Input: part model. Units: mm. Frame: model coordinates. Face numbers are marked on the shaded views. A direction names the side the tool comes from. Coordinates: 2 decimals unless noted, no trailing zeros. Write each loop counter-clockwise with the first axis right and the second up, starting at its lowest first coordinate (ties: lowest second). Pieces come first, ordered by that corner, then holes. Notation, with made-up numbers: M 59,62.5 L 74,62.5 A30 ccw 74,91.5 Z; hole C 17,46.5 d8. An arc over 180 degrees is marked long. Use one line per item in the form item = value.
from build123d import *

# Parameters (mm, degrees)
SKETCH_1_R          = 4
EXTRUDE_1_DEPTH     = 5.5
SKETCH_2_R          = 5
EXTRUDE_2_DEPTH     = 1.5
SKETCH_3_R          = 2.75
CUT_EXTRUDE_1_DEPTH = 2
SKETCH_4_R          = 1.5
CUT_EXTRUDE_2_DEPTH = 8
CHAMFER_1_SIZE      = 0.2
CHAMFER_2_SIZE      = 0.2
CHAMFER_3_SIZE      = 0.2
CHAMFER_4_SIZE      = 0.5


with BuildPart() as part:
    # 草图1 → 拉伸1 (new body)
    with BuildSketch(Plane.XY):
        Circle(SKETCH_1_R)
    extrude(amount=EXTRUDE_1_DEPTH)

    # 草图2 → 拉伸2 (add)
    with BuildSketch(Plane.XY.offset(5.5)):
        Circle(SKETCH_2_R)
    extrude(amount=EXTRUDE_2_DEPTH)

    # 草图3 → 切除-拉伸1 (cut)
    with BuildSketch(Plane.XY.offset(7)):
        Circle(SKETCH_3_R)
    extrude(amount=-CUT_EXTRUDE_1_DEPTH, mode=Mode.SUBTRACT)

    # 草图4 → 切除-拉伸2 (cut, through all)
    with BuildSketch(Plane(origin=(0, 0, 0), x_dir=(-1, 0, 0), z_dir=(0, 0, -1))):
        Circle(SKETCH_4_R)
    extrude(amount=-CUT_EXTRUDE_2_DEPTH, mode=Mode.SUBTRACT)

    # 倒角1
    chamfer_1_edges = [part.edges().sort_by_distance(p)[0] for p in [
        (-5, 0, 5.5),
        (-5, 0, 7),
    ]]
    chamfer(chamfer_1_edges, length=CHAMFER_1_SIZE)

    # 倒角2
    chamfer_2_edges = [part.edges().sort_by_distance(p)[0] for p in [
        (-4, 0, 0),
    ]]
    chamfer(chamfer_2_edges, length=CHAMFER_2_SIZE)

    # 倒角3
    chamfer_3_edges = [part.edges().sort_by_distance(p)[0] for p in [
        (-2.75, 0, 7),
    ]]
    chamfer(chamfer_3_edges, length=CHAMFER_3_SIZE)

    # 倒角4
    chamfer_4_edges = [part.edges().sort_by_distance(p)[0] for p in [
        (1.5, 0, 5),
        (1.5, 0, 0),
    ]]
    chamfer(chamfer_4_edges, length=CHAMFER_4_SIZE)


solid = part.part
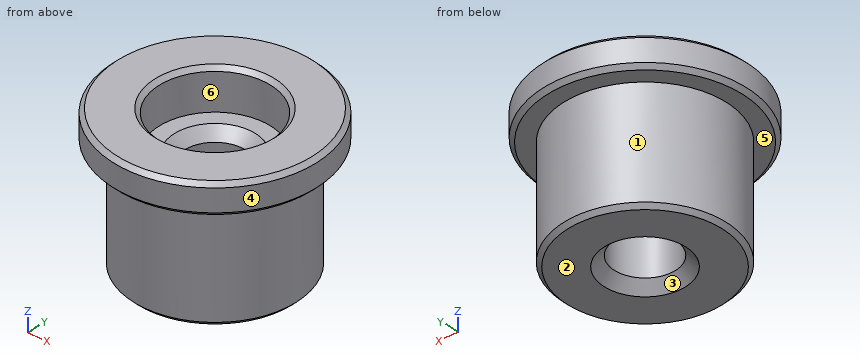
(1) Pull-direction query (X, two-part tool) for the marked faces 1, 2 and 3; classes: pulls with the +X half, pulls with the -X half, needs draft (parallel to the pull), parting line crosses it, or undercut.
Computed:
face_1 = parting line crosses it
face_2 = needs draft
face_3 = undercut
(2) Section query A-A on y = 0. Return the cut outline in (x, z), plus the area to 3 significant figures.
Computed:
outline = M -5,5.7 L -4.8,5.5 L -4,5.5 L -4,0.2 L -3.8,0 L -2,0 L -1.5,0.5 L -1.5,4.5 L -2,5 L -2.75,5 L -2.75,6.8 L -2.95,7 L -4.8,7 L -5,6.8 Z; M 1.5,0.5 L 2,0 L 3.8,0 L 4,0.2 L 4,5.5 L 4.8,5.5 L 5,5.7 L 5,6.8 L 4.8,7 L 2.95,7 L 2.75,6.8 L 2.75,5 L 2,5 L 1.5,4.5 Z
area = 32.3 mm^2
(3) Line query: probe 1 along Y at (x, z) = (0, 5.9); probe 2 along Y at (x, z) = (0, 2.55); probe 3 along Z at (x, y) = (-1.5, -1.75). Output: solid intervals per line, ascending.
Computed:
probe_1 = -5 to -2.75, 2.75 to 5
probe_2 = -4 to -1.5, 1.5 to 4
probe_3 = 0 to 5
(4) Section query C-C on z = 4. Return the cut outline in (x, y), plus the area to 3 significant figures.
Computed:
outline = C 0,0 d8; hole C 0,0 d3
area = 43.2 mm^2
(5) Set-up query: the marked faces 4, 5 and 6. Return all of +Z, -Z, +X, -X, +Y, -Y with unobstructed straight access to the full face (end or side cutting, diameter ignored); none if empty.
Computed:
face_4 = +Z, -Z
face_5 = -Z
face_6 = +Z
(6) First-contact query: pin 1 Ø2 at (x, y) = (-0.5, -0.5) entering from +Z; pin 2 Ø2.5 at (x, y) = (0, 0) entering from -Z. Flat tips, straight axial feed; report the tip coordinate or a pass-through.
Computed:
pin_1 = 4.71
pin_2 = through
